For this review, use the dimensioned drawing (mm, ordinates from the lowest corner) and the shaded views. Coordinates: 2 decimals unless noted, no trailing zeros. Loops run counter-clockwise (first coordinate to the right, second up) from the corner with the lowest first, then second, coordinate; pieces in that order, holes last. Notation, with made-up numbers: (52.5, 54.5) - (78.5, 54.5) arc R21 ccw to (78.5, 87.5) - close; hole circle Ø7 at (89, 82.5). An arc over 180 degrees is marked (long way). Answer in a Markdown table with one row per item. Add a question column.
(1) We need section A-A, the plane x = 25.4. Write out the cut boundary in (y, z) (1 decimal).
(2) We need section D-D, the plane y = 12.7. Write out the cut boundary in (x, z) (1 decimal).
(3) We need section C-C, the plane y = 24. Write out the cut boundary in (x, z) (1 decimal), plus the area to 4 significant figures.
(4) To check wall thickness, follow L1, parallel to Z at x = 88.9, y = 10 (1 decimal); L2, parallel to X at y = 20.25, z = 16.5; L3, parallel to Z at x = 27, y = 11.25 (1 decimal). State the ranges of each line that lie inside material, in increasing order. Write a range as [from, to].
(5) The part is to be moulded in two halves that separate along X. For the marked faces 1, 2 and 3, say which applies: released by +X, released by -X, zero draft, split by the parting line, or undercut.
(6) We need section B-B, the plane x = 88.9. Write out the cut boundary in (y, z) (1 decimal).
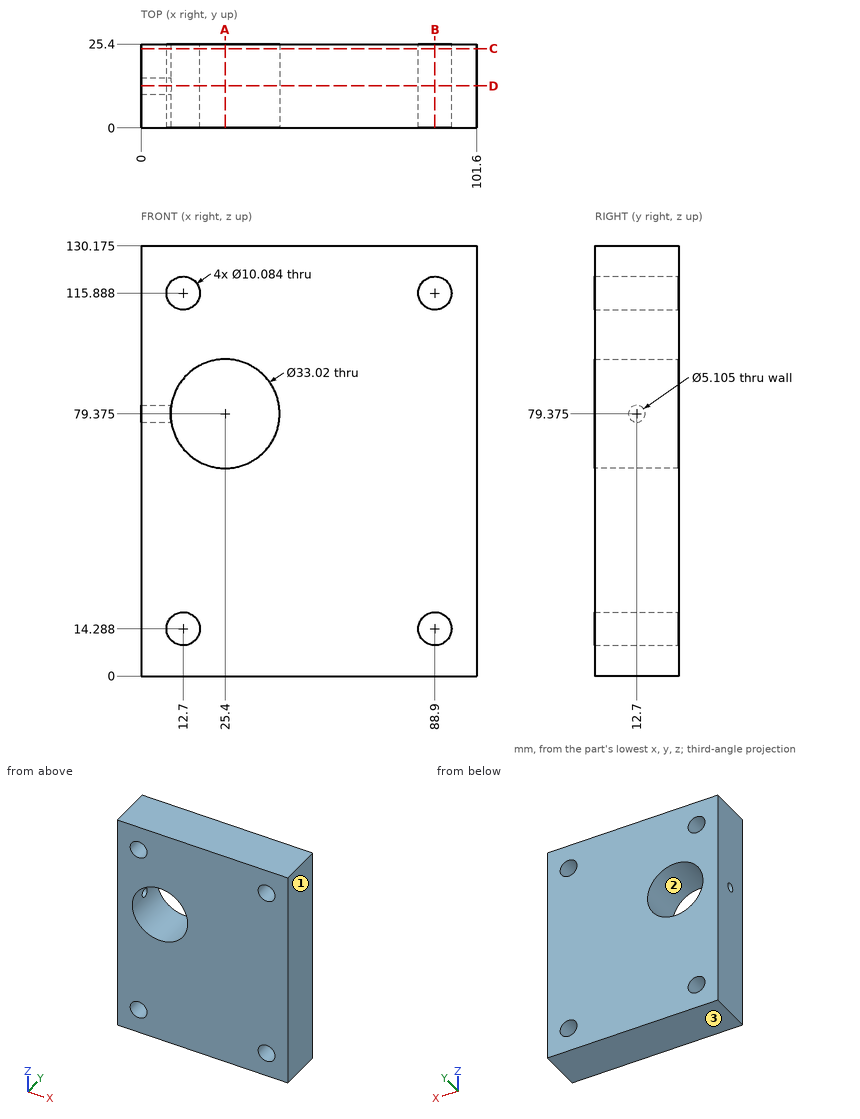
Responses:
| question | item | result |
|---|---|---|
| 1 | outline | (0, 0) - (25.4, 0) - (25.4, 62.9) - (0, 62.9) - close; (0, 95.9) - (25.4, 95.9) - (25.4, 130.2) - (0, 130.2) - close |
| 2 | outline | (0, 0) - (101.6, 0) - (101.6, 130.2) - (0, 130.2) - (0, 81.9) - (9.1, 81.9) arc R16.5 cw (long way) to (9.1, 76.8) - (0, 76.8) - close; hole circle Ø10.1 at (12.7, 14.3); hole circle Ø10.1 at (12.7, 115.9); hole circle Ø10.1 at (88.9, 14.3); hole circle Ø10.1 at (88.9, 115.9) |
| 3 | outline | (0, 0) - (101.6, 0) - (101.6, 130.2) - (0, 130.2) - close; hole circle Ø10.1 at (12.7, 14.3); hole circle Ø10.1 at (12.7, 115.9); hole circle Ø33 at (25.4, 79.4); hole circle Ø10.1 at (88.9, 14.3); hole circle Ø10.1 at (88.9, 115.9) |
| 3 | area | 12,050 mm2 |
| 4 | L1 | z = [0, 9.2], [19.3, 110.8], [120.9, 130.2] |
| 4 | L2 | x = [0, 8.17], [17.23, 84.37], [93.43, 101.6] |
| 4 | L3 | z = [0, 62.9], [95.8, 130.2] |
| 5 | face 1 | released by +X |
| 5 | face 2 | undercut |
| 5 | face 3 | zero draft |
| 6 | outline | (0, 0) - (25.4, 0) - (25.4, 9.2) - (0, 9.2) - close; (0, 19.3) - (25.4, 19.3) - (25.4, 110.8) - (0, 110.8) - close; (0, 120.9) - (25.4, 120.9) - (25.4, 130.2) - (0, 130.2) - close |
